from build123d import *
from build123d.topology import SkipClean

# Parameters (mm, degrees)
SKETCH2_R                = 60
BOSS_EXTRUDE1_DEPTH      = 60
SKETCH3_W                = 10
SKETCH3_H                = 10.47851478
BOSS_EXTRUDE2_DEPTH      = 60
FILLET2_R                = 3
CIRPATTERN1_COUNT        = 18
FILLET2_OF_CIRPATTERN1_R = 3
SKETCH4_R                = 10
CUT_EXTRUDE1_DEPTH       = 60
SKETCH5_R                = 22.481820488
BOSS_EXTRUDE3_DEPTH      = 60
SKETCH6_R                = 12.5
CUT_EXTRUDE2_DEPTH       = 12
CUT_EXTRUDE3_DEPTH       = 30.5


with BuildPart() as part:
    # Sketch2 → Boss-Extrude1 (new body)
    with BuildSketch(Plane.XY):
        Circle(SKETCH2_R)
    extrude(amount=BOSS_EXTRUDE1_DEPTH)

    # Sketch3 → Boss-Extrude2 (add)
    with BuildSketch(Plane.XY.offset(60)):
        with Locations((0, 64.76074261)):
            Rectangle(SKETCH3_W, SKETCH3_H)
    boss_extrude2 = extrude(amount=-BOSS_EXTRUDE2_DEPTH)

    # Fillet2
    fillet2_edges = [part.edges().sort_by_distance(p)[0] for p in [
        (5, 70, 30),
        (0, 70, 0),
        (-5, 70, 30),
        (0, 70, 60),
    ]]
    fillet(fillet2_edges, radius=FILLET2_R)

    # CirPattern1: Boss-Extrude2 ×18 about axis
    cirpattern1_axis = Axis((0, 0, 0), (0, 0, 1))
    for i in range(1, CIRPATTERN1_COUNT):
        add(boss_extrude2.rotate(cirpattern1_axis, i * 360 / CIRPATTERN1_COUNT))

    # Fillet2 of CirPattern1
    fillet2_of_cirpattern1_edges = [part.edges().sort_by_distance(p)[0] for p in [
        (-19.242946929, 67.488584172, 30),
        (-23.941410033, 65.778483455, 0),
        (-28.639873137, 64.068382738, 30),
        (-23.941410033, 65.778483455, 60),
        (-41.164910462, 56.837049067, 30),
        (-44.995132678, 53.623111018, 0),
        (-48.825354894, 50.40917297, 30),
        (-44.995132678, 53.623111018, 60),
        (-58.121778265, 39.330127019, 30),
        (-60.621778265, 35, 0),
        (-63.121778265, 30.669872981, 30),
        (-60.621778265, 35, 60),
        (-68.068301823, 17.079411202, 30),
        (-68.936542711, 12.155372437, 0),
        (-69.804783599, 7.231333672, 30),
        (-68.936542711, 12.155372437, 60),
        (-69.804783599, -7.231333672, 30),
        (-68.936542711, -12.155372437, 0),
        (-68.068301823, -17.079411202, 30),
        (-68.936542711, -12.155372437, 60),
        (-63.121778265, -30.669872981, 30),
        (-60.621778265, -35, 0),
        (-58.121778265, -39.330127019, 30),
        (-60.621778265, -35, 60),
        (-48.825354894, -50.40917297, 30),
        (-44.995132678, -53.623111018, 0),
        (-41.164910462, -56.837049067, 30),
        (-44.995132678, -53.623111018, 60),
        (-28.639873137, -64.068382738, 30),
        (-23.941410033, -65.778483455, 0),
        (-19.242946929, -67.488584172, 30),
        (-23.941410033, -65.778483455, 60),
        (-5, -70, 30),
        (0, -70, 0),
        (5, -70, 30),
        (0, -70, 60),
        (19.242946929, -67.488584172, 30),
        (23.941410033, -65.778483455, 0),
        (28.639873137, -64.068382738, 30),
        (23.941410033, -65.778483455, 60),
        (41.164910462, -56.837049067, 30),
        (44.995132678, -53.623111018, 0),
        (48.825354894, -50.40917297, 30),
        (44.995132678, -53.623111018, 60),
        (58.121778265, -39.330127019, 30),
        (60.621778265, -35, 0),
        (63.121778265, -30.669872981, 30),
        (60.621778265, -35, 60),
        (68.068301823, -17.079411202, 30),
        (68.936542711, -12.155372437, 0),
        (69.804783599, -7.231333672, 30),
        (68.936542711, -12.155372437, 60),
        (69.804783599, 7.231333672, 30),
        (68.936542711, 12.155372437, 0),
        (68.068301823, 17.079411202, 30),
        (68.936542711, 12.155372437, 60),
        (63.121778265, 30.669872981, 30),
        (60.621778265, 35, 0),
        (58.121778265, 39.330127019, 30),
        (60.621778265, 35, 60),
        (48.825354894, 50.40917297, 30),
        (44.995132678, 53.623111018, 0),
        (41.164910462, 56.837049067, 30),
        (44.995132678, 53.623111018, 60),
        (28.639873137, 64.068382738, 30),
        (23.941410033, 65.778483455, 0),
        (19.242946929, 67.488584172, 30),
        (23.941410033, 65.778483455, 60),
    ]]
    fillet(fillet2_of_cirpattern1_edges, radius=FILLET2_OF_CIRPATTERN1_R)

    # Sketch4 → Cut-Extrude1 (cut)
    with BuildSketch(Plane.XY.offset(60)):
        Circle(SKETCH4_R)
    extrude(amount=-CUT_EXTRUDE1_DEPTH, mode=Mode.SUBTRACT)

    # Sketch5 → Boss-Extrude3 (add)
    with BuildSketch(Plane.XY.offset(60)):
        Circle(SKETCH5_R)
    extrude(amount=-BOSS_EXTRUDE3_DEPTH)

    # Sketch6 → Cut-Extrude2 (cut)
    with BuildSketch(Plane.XY.offset(60)):
        Circle(SKETCH6_R)
    extrude(amount=-CUT_EXTRUDE2_DEPTH, mode=Mode.SUBTRACT)

    # Sketch7 → Cut-Extrude3 (cut)
    with SkipClean():  # the faces are left unmerged after this step: merging them gives an invalid solid
        with BuildSketch(Plane.XY.offset(48)):
            with BuildLine():
                Line((10.037305415, -7.45), (-10.037305415, -7.45))
                ThreePointArc((-10.037305415, -7.45), (-12.5, 0), (-10.037305415, 7.45))
                Line((-10.037305415, 7.45), (10.037305415, 7.45))
                ThreePointArc((10.037305415, 7.45), (12.5, 0), (10.037305415, -7.45))
            make_face()
        extrude(amount=-CUT_EXTRUDE3_DEPTH, mode=Mode.SUBTRACT)


solid = part.part
Build history of the part. All positions in model axes, mm. A direction names the side the tool comes from. Round coordinates to 2 decimals unless told otherwise and drop trailing zeros. Loops run counter-clockwise (first coordinate to the right, second up) from the corner with the lowest first, then second, coordinate; pieces in that order, holes last. Notation, with made-up numbers: (72.5, -23) -> (126.5, -23) arc R23 cw to (126.5, -14) -> close; hole circle Ø9 at (5, 78.25). An arc over 180 degrees is marked (long way). Answer in a Markdown table with one row per item.
Item 1: Saw through at C-C (y = 22). Write the cut outline in (x, z), and give its area (3 significant figures).
Answers below:
| item | result |
|---|---|
| outline | (-55.82, 0) -> (55.82, 0) -> (55.82, 60) -> (-55.82, 60) -> close |
| area | 6,700 mm² |
Item 2: Which spindle directions (+Z, -Z, +X, -X, +Y, -Y) get a long thin tool onto all of the face, cutting with end or side? Do faces 1 (the flat face through (-26.36, -57.81, 30.42)), 2 (the cylindrical face through (-59.525, -34.286, 0.524)), 3 (the flat face through (57.359, 27.342, 30.42)). Say none if no direction does.
Answers below:
| item | result |
|---|---|
| face 1 | +Z, -Z |
| face 2 | -Z, -X, -Y |
| face 3 | +Z, -Z, +X |
Item 3: Saw through at D-D (x = -37). Write the cut outline in (y, z), and give its area (3 significant figures).
Answers below:
| item | result |
|---|---|
| outline | (-51.87, 0) -> (51.87, 0) -> (51.87, 60) -> (-51.87, 60) -> close |
| area | 6,220 mm² |
Item 4: Pin check, flat tips, straight feed: pin 1 (2 mm diameter, centred on y = 24.5, z = 16.5, fed in from +X); pin 2 (5 mm diameter, centred on y = -25, z = 44.5, fed in from -X); pin 3 (4.5 mm diameter, centred on x = 5.5, y = 3, fed in from +Z). Stop position of each tip, or through.
Answers below:
| item | result |
|---|---|
| pin 1 | stops at x = 55.21 |
| pin 2 | stops at x = -57.63 |
| pin 3 | stops at z = 17.5 |
Item 5: Saw through at A-A (y = 0). Write the cut outline in (x, z), and give its area (3 significant figures).
Answers below:
| item | result |
|---|---|
| outline | (-60, 0) -> (60, 0) -> (60, 60) -> (12.5, 60) -> (12.5, 17.5) -> (-12.5, 17.5) -> (-12.5, 60) -> (-60, 60) -> close |
| area | 6,140 mm² |
Item 6: Saw through at B-B (x = 0). Write the cut outline in (y, z), and give its area (3 significant figures).
Answers below:
| item | result |
|---|---|
| outline | (-70, 3) arc R3 ccw to (-67, 0) -> (67, 0) arc R3 ccw to (70, 3) -> (70, 57) arc R3 ccw to (67, 60) -> (12.5, 60) -> (12.5, 48) -> (7.45, 48) -> (7.45, 17.5) -> (-7.45, 17.5) -> (-7.45, 48) -> (-12.5, 48) -> (-12.5, 60) -> (-67, 60) arc R3 ccw to (-70, 57) -> close |
| area | 7,640 mm² |
Item 7: Mould opens along X. For faces 4 (the flat face through (-63.251, -6.076, 30.42)), 5 (the cylindrical face through (30.07, 51.92, 29.58)), 6 (the flat face through (0, 70, 30)) say: +X half, -X half, draft (parallel to the pull), parting line (faces both ways), or undercut.
Answers below:
| item | result |
|---|---|
| face 4 | -X half |
| face 5 | undercut |
| face 6 | draft |
Item 8: Drill centre lines: L1, parallel to Y at x = 0, z = 56; L2, parallel to X at y = 0, z = 54.25; L3, parallel to Y at x = 42.5, z = 56.5. Where is each one in solid material? Low to high. Write a range as [from, to].
Answers below:
| item | result |
|---|---|
| L1 | y = [-70, -12.5], [12.5, 70] |
| L2 | x = [-60, -12.5], [12.5, 60] |
| L3 | y = [-55.45, -42.87], [-42.35, 42.35], [42.87, 55.45] |
